The model under review builds one solid part; all positions refer to its coordinate system, in mm. Face numbers are marked on the shaded views. A direction names the side the tool comes from. Coordinates: 2 decimals unless noted, no trailing zeros. Write each loop counter-clockwise with the first axis right and the second up, starting at its lowest first coordinate (ties: lowest second). Pieces come first, ordered by that corner, then holes. Notation, with made-up numbers: (18, 3.5) - (72, 3.5) arc R23 cw to (72, 34.5) - close; hole circle Ø6 at (-21.5, 84). An arc over 180 degrees is marked (long way). Use one line per item in the form item = value. Start each with the question number.
```python
from build123d import *

# Parameters (mm, degrees)
SKETCH1_R           = 7.5
BOSS_EXTRUDE6_DEPTH = 6
BOSS_EXTRUDE7_DEPTH = 21
SKETCH4_R           = 2.65
CUT_EXTRUDE7_DEPTH  = 6
SKETCH7_R           = 3
CUT_EXTRUDE8_DEPTH  = 0.77
SKETCH8_R           = 2.3
CUT_EXTRUDE9_DEPTH  = 6


with BuildPart() as part:
    # Sketch1 → Boss-Extrude6 (new body)
    with BuildSketch(Plane(origin=(0, 0, 0), x_dir=(1, 0, 0), z_dir=(0, 1, 0))):
        Circle(SKETCH1_R)
    extrude(amount=BOSS_EXTRUDE6_DEPTH)

    # Sketch1<9> → Boss-Extrude7 (add)
    with BuildSketch(Plane(origin=(0, 0, 0), x_dir=(1, 0, 0), z_dir=(0, 1, 0))):
        with BuildLine():
            ThreePointArc((7.5, 0), (7.341797347, 1.532322328), (6.873863542, 3))
            Line((6.873863542, 3), (-6.873863542, 3))
            ThreePointArc((-6.873863542, 3), (-7.5, 0), (-6.873863542, -3))
            Line((-6.873863542, -3), (6.873863542, -3))
            ThreePointArc((6.873863542, -3), (7.341797347, -1.532322328), (7.5, 0))
        make_face()
    extrude(amount=BOSS_EXTRUDE7_DEPTH)

    # Sketch4 → Cut-Extrude7 (cut)
    with BuildSketch(Plane.XY.offset(3)):
        with Locations((0, 13.5)):
            Circle(SKETCH4_R)
    extrude(amount=-CUT_EXTRUDE7_DEPTH, mode=Mode.SUBTRACT)

    # Sketch7 → Cut-Extrude8 (cut)
    with BuildSketch(Plane.XY.offset(3)):
        with Locations((0, 13.5)):
            Circle(SKETCH7_R)
    extrude(amount=-CUT_EXTRUDE8_DEPTH, mode=Mode.SUBTRACT)

    # Sketch8 → Cut-Extrude9 (cut)
    with BuildSketch(Plane.XZ):
        Circle(SKETCH8_R)
    extrude(amount=-CUT_EXTRUDE9_DEPTH, mode=Mode.SUBTRACT)


solid = part.part
```
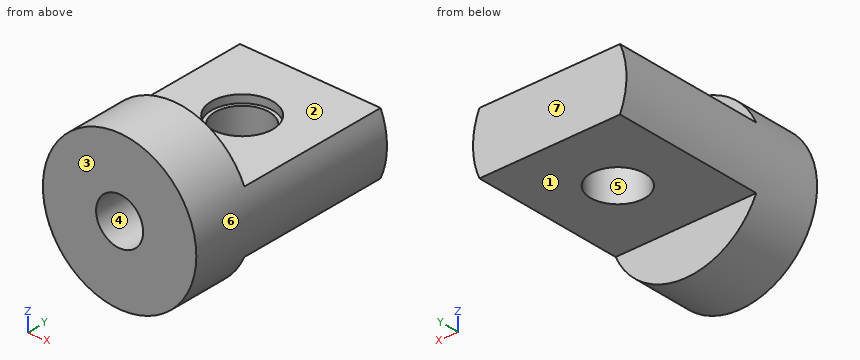
1. For L1, parallel to Z at x = 0, y = 2.7; L2, parallel to Y at x = 0, z = 2.45; L3, parallel to Y at x = -2.25, z = 6.25, list the stretches that pass through material, from the lowest coordinate up.
2. The part is to be moulded in two halves that separate along X. For the marked faces 4, 5, 6 and 7, say which applies: released by +X, released by -X, zero draft, split by the parting line, or undercut.
3. Take a section at D-D (z = -1). State the section outline as (x, y) points.
4. For the marked faces 1, 2 and 3, list the 3-axis set-ups (+Z, -Z, +X, -X, +Y, -Y) from which the entire face can be reached by the end or side of a thin tool; tool diameter is ignored.
5. For P1, Ø7, axis at x = -2, y = 11.5, coming from the +Z side; P2, Ø1, axis at x = -5.5, y = 8.5, coming from the -Z side; P3, Ø3.5, axis at x = 0, z = 0, coming from the -Y side, all flat-tipped, find the tip position at first contact; note any pin that passes through.
6. Take a section at B-B (x = 0). State the section outline as (y, z) points.
7. Take a section at A-A (y = 13.5). State the section outline as (x, z) points.
8. Take a section at C-C (x = -6). State the section outline as (y, z) points, plus the area to 3 significant figures.
Returned:
q1.L1 = -7.5 to -2.3, 2.3 to 7.5
q1.L2 = 0 to 10.5, 16.5 to 21
q1.L3 = 0 to 6
q2.face_4 = undercut
q2.face_5 = undercut
q2.face_6 = split by the parting line
q2.face_7 = zero draft
q3.outline = (-7.43, 0) - (-2.07, 0) - (-2.07, 6) - (2.07, 6) - (2.07, 0) - (7.43, 0) - (7.43, 21) - (-7.43, 21) - close; hole circle Ø5.3 at (0, 13.5)
q4.face_1 = -Z, +X, -X, +Y
q4.face_2 = +Z, +X, -X, +Y
q4.face_3 = +Z, -Z, +X, -X, -Y
q5.P1 = 3
q5.P2 = -3
q5.P3 = 6
q6.outline = (0, -7.5) - (6, -7.5) - (6, -3) - (10.85, -3) - (10.85, 2.23) - (10.5, 2.23) - (10.5, 3) - (6, 3) - (6, 7.5) - (0, 7.5) - (0, 2.3) - (6, 2.3) - (6, -2.3) - (0, -2.3) - close; (16.15, -3) - (21, -3) - (21, 3) - (16.5, 3) - (16.5, 2.23) - (16.15, 2.23) - close
q7.outline = (-6.87, -3) - (-2.65, -3) - (-2.65, 2.23) - (-3, 2.23) - (-3, 3) - (-6.87, 3) arc R7.5 ccw to start; (2.65, -3) - (6.87, -3) arc R7.5 ccw to (6.87, 3) - (3, 3) - (3, 2.23) - (2.65, 2.23) - close
q8.outline = (0, -4.5) - (6, -4.5) - (6, -3) - (21, -3) - (21, 3) - (6, 3) - (6, 4.5) - (0, 4.5) - close
q8.area = 144 mm²
